```python
from build123d import *

# Parameters (mm, degrees)
CABFRONTOUTLINE_W               = 628.65
CABFRONTOUTLINE_H               = 396.08125
CABFRONT_THICKNESS_DEPTH        = 17.78
CABFRONT_COINDOORCUTS_R         = 1.5875
CABFRONT_COINDOORCUTS_R_2       = 15.08125
CABFRONT_COINDOORCUTS_R_3       = 3.4925
CABFRONT_COINDOORCUTS_W         = 308.0004
CABFRONT_COINDOORCUTS_H         = 261.9629
CUT_EXTRUDE1_DEPTH              = 17.78
CABFRONTBOTTOMLEDGE_DEPTH_DEPTH = 5.08
CUT_EXTRUDE4_DEPTH              = 396.08125
FILLET1_R                       = 20.6502
SKETCH2_R                       = 4.7625
CUT_EXTRUDE5_DEPTH              = 76.2
SKETCH3_R                       = 4.7625
CUT_EXTRUDE6_DEPTH              = 76.2
SKETCH4_R                       = 4.7625
CUT_EXTRUDE7_DEPTH              = 76.2


with BuildPart() as part:
    # CabFrontOutline → CabFront_Thickness (new body)
    with BuildSketch(Plane.XY):
        with Locations((12009.966666666, -5854.303125)):
            Rectangle(CABFRONTOUTLINE_W, CABFRONTOUTLINE_H)
    extrude(amount=-CABFRONT_THICKNESS_DEPTH)

    # CabFront_CoinDoorCuts → Cut-Extrude1 (cut)
    with BuildSketch(Plane.XY):
        with Locations((11753.109166666, -5893.59375)):
            Circle(CABFRONT_COINDOORCUTS_R)
        with Locations((11753.109166666, -5950.74375)):
            Circle(CABFRONT_COINDOORCUTS_R)
        with Locations((12266.824166666, -5893.59375)):
            Circle(CABFRONT_COINDOORCUTS_R)
        with Locations((12266.824166666, -5950.74375)):
            Circle(CABFRONT_COINDOORCUTS_R)
        with Locations((12266.824166666, -5836.44375)):
            Circle(CABFRONT_COINDOORCUTS_R)
        with Locations((12267.141666666, -5761.0375)):
            Circle(CABFRONT_COINDOORCUTS_R_2)
        with Locations((12173.479166666, -5831.68125)):
            Circle(CABFRONT_COINDOORCUTS_R_3)
        with Locations((12266.824166666, -5865.01875)):
            Circle(CABFRONT_COINDOORCUTS_R)
        with Locations((12266.824166666, -5922.16875)):
            Circle(CABFRONT_COINDOORCUTS_R)
        with Locations((12266.824166666, -5979.31875)):
            Circle(CABFRONT_COINDOORCUTS_R)
        with Locations((12209.991666666, -6037.10375)):
            Circle(CABFRONT_COINDOORCUTS_R)
        with Locations((12009.966666666, -6037.10375)):
            Circle(CABFRONT_COINDOORCUTS_R)
        with Locations((11809.941666666, -6037.10375)):
            Circle(CABFRONT_COINDOORCUTS_R)
        with Locations((11753.109166666, -5979.31875)):
            Circle(CABFRONT_COINDOORCUTS_R)
        with Locations((11753.109166666, -5922.16875)):
            Circle(CABFRONT_COINDOORCUTS_R)
        with Locations((11753.109166666, -5865.01875)):
            Circle(CABFRONT_COINDOORCUTS_R)
        with Locations((11846.454166666, -5831.68125)):
            Circle(CABFRONT_COINDOORCUTS_R_3)
        with Locations((12009.966666666, -5972.175)):
            Circle(CABFRONT_COINDOORCUTS_R_3)
        with Locations((12009.966666666, -5691.1875)):
            Circle(CABFRONT_COINDOORCUTS_R_3)
        with Locations((12009.966666666, -5831.68125)):
            Rectangle(CABFRONT_COINDOORCUTS_W, CABFRONT_COINDOORCUTS_H)
        with BuildLine():
            Line((11734.654409808, -5693.754968556), (11739.23011943, -5693.754968556))
            ThreePointArc((11739.23011943, -5693.754968556), (11748.029166666, -5687.976468556), (11756.828213901, -5693.754968556))
            Line((11756.828213901, -5693.754968556), (11761.386355753, -5693.754968556))
            ThreePointArc((11761.386355753, -5693.754968556), (11767.531113043, -5692.357368906), (11771.079666666, -5697.564968556))
            ThreePointArc((11771.079666666, -5697.564968556), (11767.531113043, -5702.772568206), (11761.386355753, -5701.374968556))
            Line((11761.386355753, -5701.374968556), (11756.828213901, -5701.374968556))
            ThreePointArc((11756.828213901, -5701.374968556), (11754.760305425, -5704.393665595), (11751.712166666, -5706.417925308))
            Line((11751.712166666, -5706.417925308), (11751.712166666, -5721.30243896))
            ThreePointArc((11751.712166666, -5721.30243896), (11748.029166666, -5731.092968556), (11744.346166666, -5721.30243896))
            Line((11744.346166666, -5721.30243896), (11744.346166666, -5706.417925308))
            ThreePointArc((11744.346166666, -5706.417925308), (11741.298027907, -5704.393665595), (11739.23011943, -5701.374968556))
            Line((11739.23011943, -5701.374968556), (11734.654409809, -5701.374968556))
            ThreePointArc((11734.654409809, -5701.374968556), (11724.978666666, -5697.564968556), (11734.654409808, -5693.754968556))
        make_face()
    extrude(amount=-CUT_EXTRUDE1_DEPTH, mode=Mode.SUBTRACT)

    # CabFront_BottomLedge → CabFrontBottomLedge_Depth (cut)
    with BuildSketch(Plane.XY):
        Polygon((11975.041666666, -6028.21375), (11695.641666666, -6028.21375), (11695.641666666, -6045.99375), (12324.291666666, -6045.99375), (12324.291666666, -6028.21375), align=None)
    extrude(amount=-CABFRONTBOTTOMLEDGE_DEPTH_DEPTH, mode=Mode.SUBTRACT)

    # CabFront_EdgeBevel → Cut-Extrude4 (cut)
    with BuildSketch(Plane.XZ.offset(6052.34375)):
        Polygon((11701.991666666, -11.43), (11701.991666666, 0), (11695.641666666, 0), (11695.641666666, -17.78), align=None)
        Polygon((12317.941666666, -11.43), (12324.291666666, -17.78), (12324.291666666, 0), (12317.941666666, 0), align=None)
    extrude(amount=-CUT_EXTRUDE4_DEPTH, mode=Mode.SUBTRACT)

    # Fillet1
    fillet1_edges = [part.edges().sort_by_distance(p)[0] for p in [
        (11855.966466666, -5962.6627, -8.89),
        (11855.966466666, -5700.6998, -8.89),
        (12163.966866666, -5700.6998, -8.89),
        (12163.966866666, -5962.6627, -8.89),
    ]]
    fillet(fillet1_edges, radius=FILLET1_R)

    # Sketch2 → Cut-Extrude5 (cut)
    with BuildSketch(Plane(origin=(5872.794384557, 0, 5872.794384557), x_dir=(0.707106781, 0, -0.707106781), z_dir=(0.707106781, 0, 0.707106781))):
        with Locations((8282.639891397, -5922.16875)):
            Circle(SKETCH2_R)
        with Locations((8282.639891397, -5979.31875)):
            Circle(SKETCH2_R)
    extrude(amount=-CUT_EXTRUDE5_DEPTH, mode=Mode.SUBTRACT)

    # Sketch3 → Cut-Extrude6 (cut)
    with BuildSketch(Plane(origin=(6137.172282109, 0, -6137.172282109), x_dir=(0.707106781, 0, 0.707106781), z_dir=(-0.707106781, 0, 0.707106781))):
        with Locations((8702.017852251, -5922.16875)):
            Circle(SKETCH3_R)
        with Locations((8702.017852251, -5979.31875)):
            Circle(SKETCH3_R)
    extrude(amount=-CUT_EXTRUDE6_DEPTH, mode=Mode.SUBTRACT)

    # Sketch4 → Cut-Extrude7 (cut)
    with BuildSketch(Plane(origin=(6137.165932109, 0, -6137.165932109), x_dir=(0.707106781, 0, 0.707106781), z_dir=(-0.707106781, 0, 0.707106781))):
        with Locations((8702.008871995, -5950.74375)):
            Circle(SKETCH4_R)
        with Locations((8702.008871995, -5893.59375)):
            Circle(SKETCH4_R)
    extrude(amount=-CUT_EXTRUDE7_DEPTH, mode=Mode.SUBTRACT)


solid = part.part
```
Could you check a few things on this model? Use its own coordinates, in mm. A direction names the side the tool comes from. Round coordinates to 2 decimals unless told otherwise and drop trailing zeros. Loops run counter-clockwise (first coordinate to the right, second up) from the corner with the lowest first, then second, coordinate; pieces in that order, holes last. Notation, with made-up numbers: M 50.5,37.5 L 61.5,37.5 A13 ccw 61.5,58.5 Z; hole C 68,-11 d2. An arc over 180 degrees is marked long. Write item = value, one per line.
1. Thinking about a two-plate mould opening in Y: for faces 5 (the face through (12310.135, -5921.959, -10.352)), 6 (the face through (11709.474, -5981.143, -10.169)), 7 (the face through (12006, -6052.344, -9)), 8 (the face through (12006, -5964, 0)), which applies, +Y half, -Y half, draft (parallel to the pull), parting line (faces both ways), or undercut?
Results below:
face_5 = undercut
face_6 = undercut
face_7 = -Y half
face_8 = draft
2. I want a section at A-A, the plane y = -5847. Write out the boundary of the cut face in (x, z).
Results below:
outline = M 11695.64,-17.78 L 11855.97,-17.78 L 11855.97,0 L 11701.99,0 L 11701.99,-11.43 Z; M 12163.97,-17.78 L 12324.29,-17.78 L 12317.94,-11.43 L 12317.94,0 L 12163.97,0 Z
3. I want a section at B-B, the plane x = 11951. Write out the boundary of the cut face in (y, z).
Results below:
outline = M -6052.34,-17.78 L -5962.66,-17.78 L -5962.66,0 L -6028.21,0 L -6028.21,-5.08 L -6045.99,-5.08 L -6045.99,0 L -6052.34,0 Z; M -5700.7,-17.78 L -5656.26,-17.78 L -5656.26,0 L -5700.7,0 Z
4. I need wall thicknesses on probe 1 along Y at (x, z) = (11760, -3); probe 2 along Y at (x, z) = (11923.5, -3); probe 3 along Y at (x, z) = (11895.5, -9.75). Which ranges of each line are inside material? Lowest first, please.
Results below:
probe_1 = -6052.34 to -6045.99, -6028.21 to -5701.37, -5693.75 to -5656.26
probe_2 = -6052.34 to -6045.99, -6028.21 to -5962.66, -5700.7 to -5656.26
probe_3 = -6052.34 to -5962.66, -5700.7 to -5656.26
5. Will these pins go through, and if not, where does the flat tip stop? P1, Ø18, axis at x = 11748.03, y = -5725.5, coming from the +Z side; P2, Ø6, axis at y = -5794.5, z = -4, coming from the -X side; P3, Ø5.5, axis at y = -5833.5, z = -6, coming from the +X side; P4, Ø8, axis at y = -6006.5, z = -12, coming from the -X side.
Results below:
P1 = 0
P2 = 11701.99
P3 = 12317.94
P4 = 11697.42
6. I want a section at D-D, the plane z = -8.5. Count the separate pieces of the cut face and the enclosed holes in it, and give its area (3 significant figures).
Results below:
separate_pieces = 1
enclosed_holes = 21
area = 161,000 mm²
7. I want a section at C-C, the plane y = -6020. Write out the boundary of the cut face in (x, z).
Results below:
outline = M 11695.64,-17.78 L 12324.29,-17.78 L 12317.94,-11.43 L 12317.94,0 L 11701.99,0 L 11701.99,-11.43 Z
8. Which directions (+Z, -Z, +X, -X, +Y, -Y) give clear straight access to the entire face, cutting with the end or side of a thin tool? Please do faces 1 (the face through (12163.967, -5833, -9)), 2 (the face through (11701.992, -5857, -6)), 3 (the face through (12006, -6037, -5.08)), 4 (the face through (12006, -5984, -17.78)).
Results below:
face_1 = +Z, -Z
face_2 = +Z, -X, +Y, -Y
face_3 = +Z, +X, -X
face_4 = -Z, +X, -X, +Y, -Y
